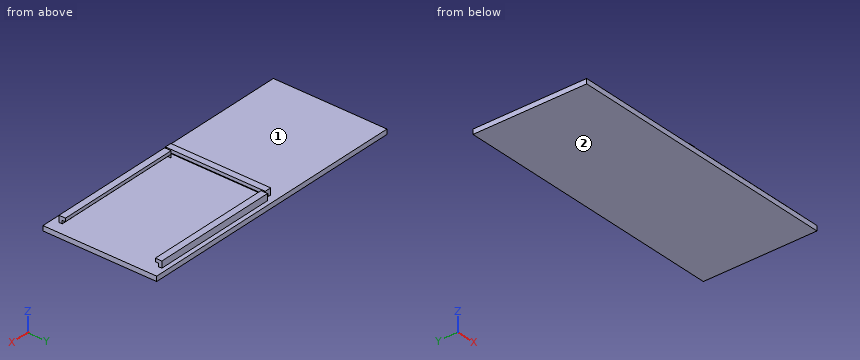
```python
from build123d import *

# Parameters (mm, degrees)
F0_W     = 4
F0_H     = 61.5
F0_W_2   = 78
F0_H_2   = 4
F1_DEPTH = 3
F2_DEPTH = 7
F3_W     = 2
F3_H     = 2
F4_DEPTH = 77.9
F5_W     = 2
F5_H     = 2
F6_DEPTH = 64.1
F7_W     = 2
F7_H     = 2
F8_DEPTH = 78


# Not quite as in the source:
# - a feature names something its author has since deleted; it is built from what else it names


with BuildPart() as f1:
    # F0 (on Top) → F1 (new body)
    with BuildSketch(Plane.XY):
        Polygon((85, 35), (-85, 35), (-85, -25.7047470659), (-85, -35), (-7, -35), (85, -35), align=None)
        with Locations((-2.7990786843, -0.482085079)):
            Rectangle(F0_W, F0_H, mode=Mode.SUBTRACT)
        with Locations((39, -28.9953801334)):
            Rectangle(F0_W_2, F0_H_2, mode=Mode.SUBTRACT)
        with Locations((39, 30.3457357436)):
            Rectangle(F0_W_2, F0_H_2, mode=Mode.SUBTRACT)
    extrude(amount=F1_DEPTH)

    # F0 (on Top) → F2 (join)
    with BuildSketch(Plane.XY):
        with Locations((-2.7990786843, -0.482085079)):
            Rectangle(F0_W, F0_H)
        with Locations((39, -28.9953801334)):
            Rectangle(F0_W_2, F0_H_2)
        with Locations((39, 30.3457357436)):
            Rectangle(F0_W_2, F0_H_2)
    extrude(amount=F2_DEPTH)

    # F3 (on face) → F4 (cut)
    with BuildSketch(Plane.YZ.offset(78)):
        with Locations((-27.9953801334, 4)):
            Rectangle(F3_W, F3_H)
    extrude(amount=-F4_DEPTH, mode=Mode.SUBTRACT)

    # F5 (on face) → F6 (cut)
    with BuildSketch(Plane.XZ.offset(31.232085079)):
        with Locations((-1.7990786843, 4)):
            Rectangle(F5_W, F5_H)
    extrude(amount=-F6_DEPTH, mode=Mode.SUBTRACT)

    # F7 (on face) → F8 (cut)
    with BuildSketch(Plane.YZ.offset(78)):
        with Locations((29.3457357436, 4)):
            Rectangle(F7_W, F7_H)
    extrude(amount=-F8_DEPTH, mode=Mode.SUBTRACT)


solid = f1.part
```
The model under review builds one solid part; all positions refer to its coordinate system, in mm. Face numbers are marked on the shaded views. Round coordinates to 2 decimals unless told otherwise and drop trailing zeros. Write each loop counter-clockwise with the first axis right and the second up, starting at its lowest first coordinate (ties: lowest second). Pieces come first, ordered by that corner, then holes.
(1) We need section C-C on x = -16. Give the boundary of the cut face in (y, z), and give its area (3 significant figures).
(2) We need section B-B on x = 59.5. Give the boundary of the cut face in (y, z).
(3) Insertion check: pin 1 (21 mm diameter, centred on x = -39.5, y = -10.5, fed in from +Z); pin 2 (1 mm diameter, centred on x = 25.5, z = 4, fed in from +Y); pin 3 (1.2 mm diameter, centred on x = -3, z = 5, fed in from -Y); pin 4 (1.6 mm diameter, centred on x = 41.5, y = -28, fed in from -Z). Each pin has a flat end and moves straight along its axis. Give the tip position at first contact, or say it passes through.
(4) We need section A-A on y = -20. Give the boundary of the cut face in (x, z), and give its area (3 significant figures).
(5) Mouldability with a two-part tool opening along Y and no side actions: class the marked faces 1 and 2 as +Y half, -Y half, draft (parallel to the pull), parting line (faces both ways), or undercut.
(6) Wall thickness on L1, parallel to Y at x = 77, z = 3.5; L2, parallel to Y at x = 21, z = 6.5; L3, parallel to Z at x = -1.5, y = 23: over which ranges is each line inside the solid? List them lowest first.
Findings below:
1. outline: (-35, 0) - (35, 0) - (35, 3) - (-35, 3) - close
1. area: 210 mm2
2. outline: (-35, 0) - (35, 0) - (35, 3) - (32.35, 3) - (32.35, 7) - (28.35, 7) - (28.35, 5) - (30.35, 5) - (30.35, 3) - (-29, 3) - (-29, 5) - (-27, 5) - (-27, 7) - (-31, 7) - (-31, 3) - (-35, 3) - close
3. pin 1: stops at z = 3
3. pin 2: stops at y = 32.35
3. pin 3: stops at y = -31.23
3. pin 4: stops at z = 0
4. outline: (-85, 0) - (85, 0) - (85, 3) - (-2.8, 3) - (-2.8, 5) - (-0.8, 5) - (-0.8, 7) - (-4.8, 7) - (-4.8, 3) - (-85, 3) - close
4. area: 522 mm2
5. face 1: undercut
5. face 2: draft
6. L1: y = -31 to -29, 30.35 to 32.35
6. L2: y = -31 to -27, 28.35 to 32.35
6. L3: z = 0 to 3, 5 to 7
